```python
from build123d import *

# Parameters (mm, degrees)
F0_W     = 100
F0_H     = 100
F0_R     = 2.25
F1_DEPTH = 3
F2_R     = 5
F3_SIZE  = 2


with BuildPart() as f1:
    # F0 (on Top) → F1 (new body)
    with BuildSketch(Plane.XY):
        with Locations((50, 50)):
            Rectangle(F0_W, F0_H)
        with Locations((5, 5)):
            Circle(F0_R, mode=Mode.SUBTRACT)
        with Locations((14, 14)):
            Circle(F0_R, mode=Mode.SUBTRACT)
        with Locations((95, 5)):
            Circle(F0_R, mode=Mode.SUBTRACT)
        with Locations((86, 14)):
            Circle(F0_R, mode=Mode.SUBTRACT)
        with Locations((14, 86)):
            Circle(F0_R, mode=Mode.SUBTRACT)
        with Locations((5, 95)):
            Circle(F0_R, mode=Mode.SUBTRACT)
        with BuildLine():
            Line((72.181073, 12), (27.818927, 12))
            ThreePointArc((27.818927, 12), (18.887302, 18.887302), (12, 27.818927))
            Line((12, 27.818927), (12, 72.181073))
            ThreePointArc((12, 72.181073), (18.887302, 81.112698), (27.818927, 88))
            Line((27.818927, 88), (72.181073, 88))
            ThreePointArc((72.181073, 88), (81.112698, 81.112698), (88, 72.181073))
            Line((88, 72.181073), (88, 27.818927))
            ThreePointArc((88, 27.818927), (81.112698, 18.887302), (72.181073, 12))
        make_face(mode=Mode.SUBTRACT)
        with Locations((86, 86)):
            Circle(F0_R, mode=Mode.SUBTRACT)
        with Locations((95, 95)):
            Circle(F0_R, mode=Mode.SUBTRACT)
    extrude(amount=F1_DEPTH)

    # F2
    f2_edges = [f1.edges().sort_by_distance(p)[0] for p in [
        (100, 0, 1.5),
        (100, 100, 1.5),
        (0, 0, 1.5),
        (0, 100, 1.5),
    ]]
    fillet(f2_edges, radius=F2_R)

    # F3
    f3_edges = [f1.edges().sort_by_distance(p)[0] for p in [
        (2.75, 95, 3),
        (2.75, 5, 3),
        (92.75, 5, 3),
        (92.75, 95, 3),
        (11.75, 86, 0),
        (11.75, 14, 0),
        (83.75, 14, 0),
        (83.75, 86, 0),
    ]]
    chamfer(f3_edges, length=F3_SIZE)


solid = f1.part
```
The listing builds one solid part. Answer for the finished solid, in the listing's coordinates (mm). A direction names the side the tool comes from. Give positions to 0.01 mm unless a question says otherwise; leave off trailing zeros. Write each loop counter-clockwise with the first axis right and the second up, starting at its lowest first coordinate (ties: lowest second). Pieces come first, ordered by that corner, then holes. Notation, with made-up numbers: (-29.75, 49.5) -> (28.25, 49.5) arc R25 cw to (28.25, 78.5) -> close; hole circle Ø2 at (40.25, -21). An arc over 180 degrees is marked (long way). Write item = value, one per line. Start each with the question number.
1) Determine the mould class of faces 1 (the face through (1, 2, 2)), 2 (the face through (94, 51, 3)), 3 (the face through (18.999, 18.776, 1.479)), 4 (the face through (4.512, 92.804, 0.493)) for opening direction Y: +Y half, -Y half, draft (parallel to the pull), parting line (faces both ways), or undercut.
2) Which of the six approach directions +Z, -Z, +X, -X, +Y, -Y give full straight-line access (tool end or side, diameter ignored) to faces 5 (the face through (49, 100, 1)), 6 (the face through (12, 50, 1))?
3) Each of these flat-tipped pins is pushed along its axis until it touches: pin 1 (7 mm diameter, centred on x = 95, y = 5, fed in from -Z); pin 2 (7 mm diameter, centred on x = 5, y = 95, fed in from +Z); pin 3 (6 mm diameter, centred on x = 86, y = 14, fed in from -Z). Where does it stop, or does it pass through?
4) The part is cut by section C-C, the plane x = 14. Determine the outline of the cut face in (y, z).
5) The part is cut by section A-A, the plane x = 57.5. Determine the outline of the cut face in (y, z), and give its area (3 significant figures).
6) Straight lines are drawn through the part: line 1 along Y through (x, z) = (95, 0.8); line 2 along Y through (x, z) = (30.5, 2.25). For each, find the intervals that lie inside material, in ascending order.
Solutions:
q1.face_1 = -Y half
q1.face_2 = draft
q1.face_3 = undercut
q1.face_4 = undercut
q2.face_5 = +Z, -Z, +X, -X, +Y
q2.face_6 = +Z, -Z
q3.pin_1 = 0
q3.pin_2 = 2.25
q3.pin_3 = 1.25
q4.outline = (0, 0) -> (9.75, 0) -> (11.75, 2) -> (11.75, 3) -> (0, 3) -> close; (16.25, 2) -> (18.25, 0) -> (24.7, 0) -> (24.7, 3) -> (16.25, 3) -> close; (75.3, 0) -> (81.75, 0) -> (83.75, 2) -> (83.75, 3) -> (75.3, 3) -> close; (88.25, 2) -> (90.25, 0) -> (100, 0) -> (100, 3) -> (88.25, 3) -> close
q5.outline = (0, 0) -> (12, 0) -> (12, 3) -> (0, 3) -> close; (88, 0) -> (100, 0) -> (100, 3) -> (88, 3) -> close
q5.area = 72.0 mm²
q6.line_1 = 0 to 2.75, 7.25 to 92.75, 97.25 to 100
q6.line_2 = 0 to 12, 88 to 100
